from build123d import *

# Parameters (mm, degrees)
SKETCH1_R               = 27.5
BOSS_EXTRUDE1_DEPTH     = 4
SKETCH2_R               = 27.5
SKETCH2_R_2             = 15
BOSS_EXTRUDE2_DEPTH     = 1
SKETCH3_R               = 3.429
CUT_EXTRUDE1_DEPTH      = 40.210967853
CUT_EXTRUDE1_DEPTH_BACK = 40.210967853
SKETCH4_R               = 12
SKETCH4_R_2             = 3.429
BOSS_EXTRUDE3_DEPTH     = 15
CHAMFER1_SIZE           = 0.5


with BuildPart() as part:
    # Sketch1 → Boss-Extrude1 (new body)
    with BuildSketch(Plane(origin=(0, 0, 0), x_dir=(0, 0, -1), z_dir=(1, 0, 0))):
        Circle(SKETCH1_R)
    extrude(amount=BOSS_EXTRUDE1_DEPTH)

    # Sketch2 → Boss-Extrude2 (add)
    with BuildSketch(Plane(origin=(4, 0, 0), x_dir=(0, 0, -1), z_dir=(1, 0, 0))):
        Circle(SKETCH2_R)
        Circle(SKETCH2_R_2, mode=Mode.SUBTRACT)
    extrude(amount=BOSS_EXTRUDE2_DEPTH)

    # Sketch3 → Cut-Extrude1 (cut, two sides)
    with BuildSketch(Plane.ZY) as cut_extrude1_sk:
        with Locations(Location((0, 0, 0), (0, 0, 180))):
            Circle(SKETCH3_R)
    extrude(amount=CUT_EXTRUDE1_DEPTH, mode=Mode.SUBTRACT)
    extrude(cut_extrude1_sk.sketch, amount=-CUT_EXTRUDE1_DEPTH_BACK, mode=Mode.SUBTRACT)

    # Sketch4 → Boss-Extrude3 (add)
    with BuildSketch(Plane(origin=(4, 0, 0), x_dir=(0, 0, -1), z_dir=(1, 0, 0))):
        Circle(SKETCH4_R)
        Circle(SKETCH4_R_2, mode=Mode.SUBTRACT)
    extrude(amount=BOSS_EXTRUDE3_DEPTH)

    # Chamfer1
    chamfer1_edges = [part.edges().sort_by_distance(p)[0] for p in [
        (5, 0, 27.5),
    ]]
    chamfer(chamfer1_edges, length=CHAMFER1_SIZE)


solid = part.part
Source: CAD feature listing. Evaluate the final solid. Frame: model axes, mm. A direction names the side the tool comes from. Round coordinates to 2 decimals unless told otherwise and drop trailing zeros. Write each loop counter-clockwise with the first axis right and the second up, starting at its lowest first coordinate (ties: lowest second). Pieces come first, ordered by that corner, then holes. Notation, with made-up numbers: M 81,-2.5 L 85,-2.5 A36 ccw 85,36.5 Z; hole C 17.25,34 d10. An arc over 180 degrees is marked long. One line per item, written item: value. Start each with the question number.
Item 1: Mould query, pull axis Y, two halves, no side actions, for faces 1 (the cylindrical face through (4.493, 0.66, 14.985)), 2 (the cylindrical face through (2.218, -26.846, 5.961)), 3 (the flat face through (0, -6, 0)). Classes: pulls with the +Y half, pulls with the -Y half, needs draft (parallel to the pull), parting line crosses it, or undercut.
Item 2: Pin query (flat end, axial travel): pin 1 (6 mm diameter, centred on x = 3, y = 6, fed in from -Z); pin 2 (3 mm diameter, centred on x = 13.5, y = 7, fed in from +Z); pin 3 (5 mm diameter, centred on x = 16.5, y = 12.5, fed in from -Z). Return the tip coordinate at first contact, or that it passes through.
Item 3: Ray query, L1, parallel to Y at x = 14.5, z = 0; L2, parallel to Y at x = 4.65, z = 0; L3, parallel to X at y = -6, z = -15.5. Return the intervals inside material, ascending. Write a range as from..to.
Item 4: Section query C-C (x = 10.5). Return the cut outline in (y, z), plus the area to 3 significant figures.
Item 5: Section query A-A (z = 0). Return the cut outline in (x, y).
Item 6: Set-up query: faces 4 (the flat face through (4, 10, 7)), 5 (the flat face through (19, 3, -2)). Return all of +Z, -Z, +X, -X, +Y, -Y with unobstructed straight access to the full face (end or side cutting, diameter ignored); none if empty.
Result set:
1. face 1: undercut
1. face 2: parting line crosses it
1. face 3: needs draft
2. pin 1: stops at z = -27.34
2. pin 2: stops at z = 10.67
2. pin 3: stops at z = -6.63
3. L1: y = -12..-3.43, 3.43..12
3. L2: y = -27.35..-15, -12..-3.43, 3.43..12, 15..27.35
3. L3: x = 0..5
4. outline: C 0,0 d24; hole C 0,0 d6.86
4. area: 415 mm²
5. outline: M 0,-27.5 L 4.5,-27.5 L 5,-27 L 5,-15 L 4,-15 L 4,-12 L 19,-12 L 19,-3.43 L 0,-3.43 Z; M 0,3.43 L 19,3.43 L 19,12 L 4,12 L 4,15 L 5,15 L 5,27 L 4.5,27.5 L 0,27.5 Z
6. face 4: +X
6. face 5: +Z, -Z, +X, +Y, -Y
